The model under review builds one solid part; all positions refer to its coordinate system, in mm. Face numbers are marked on the shaded views. A direction names the side the tool comes from. Coordinates: 2 decimals unless noted, no trailing zeros. Loops run counter-clockwise (first coordinate to the right, second up) from the corner with the lowest first, then second, coordinate; pieces in that order, holes last. Notation, with made-up numbers: (80.25, 6) - (104.25, 6) arc R12 ccw to (104.25, 19) - close; hole circle Ø11 at (85, 54.25). An arc over 180 degrees is marked (long way). Use a Markdown table: item, result. Add a question column.
1) Add section D-D, the plane y = -65. Give the boundary of the cut face in (x, z).
2) The part is to be moulded in two halves that separate along Y. For the marked faces 1 and 2, say which applies: pulls with the +Y half, pulls with the -Y half, needs draft (parallel to the pull), parting line crosses it, or undercut.
3) To check wall thickness, follow L1, parallel to X at y = -77, z = -9.5; L2, parallel to Y at x = 200.5, z = -22; L3, parallel to Z at x = 25.5, y = -34.5. State the ranges of each line that lie inside material, in increasing order. Write a range as [from, to].
4) Clearance check with flat-ended pins moving along their axes: pin 1 (4 mm diameter, centred on x = 133.5, y = -2.5, fed in from -Z); pin 2 (3 mm diameter, centred on x = 21.5, y = -86.5, fed in from -Z); pin 3 (6 mm diameter, centred on x = 222.5, z = -70.5, fed in from +Y). State where each tip first meets the part, or that it passes through.
5) Add section C-C, the plane y = 85. Give the boundary of the cut face in (x, z).
6) Add section B-B, the plane x = 81. Give the boundary of the cut face in (y, z).
7) Add section A-A, the plane y = 0. Give the boundary of the cut face in (x, z).
8) For the marked faces 3 and 4, list the 3-axis set-ups (+Z, -Z, +X, -X, +Y, -Y) from which the entire face can be reached by the end or side of a thin tool; tool diameter is ignored.
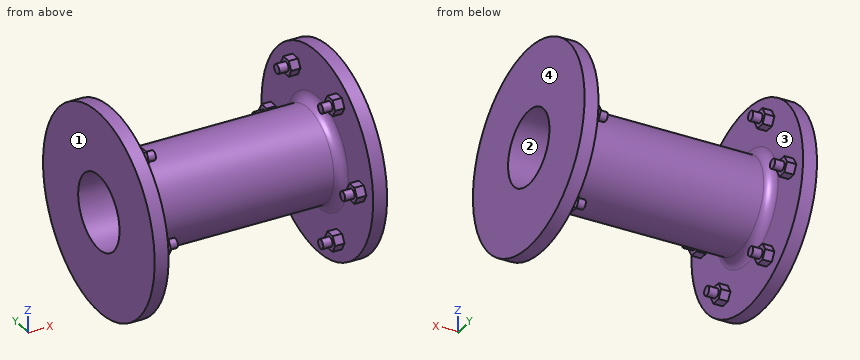
Autodesk Inventor part; units mm, degrees
ref_plane "YZ Plane" through (0, 0, 0) normal (1, 0, 0) x (0, 1, 0)
ref_plane "XZ Plane" through (0, 0, 0) normal (0, 1, 0) x (-1, 0, 0)
ref_plane "XY Plane" through (0, 0, 0) normal (0, 0, 1) x (1, 0, 0)
sketch "Skizze1" plane through (0, 0, 0) normal (1, 0, 0) x (0, 1, 0)
  circle A0 centre (0, 0) radius 40
  circle A1 centre (0, 0) radius 108
  dimension "d0" = 216
  dimension "d1" = 80
extrude "Extrusion1" add sketch "Skizze1" along normal blind 15
sketch "Skizze2" plane through (15, 0, 0) normal (1, 0, 0) x (0, 0, -1)
  circle A0 centre (0, 0) radius 40
  circle A1 centre (0, 0) radius 50
  dimension "d4" = 100
extrude "Extrusion2" add sketch "Skizze2" along normal blind 110
fillet "Rundung1" radius 10 1 edges at (15, 0, 50)
sketch "Skizze3" plane through (15, 0, 0) normal (1, 0, 0) x (0, 0, -1)
  circle A0 centre (0, -85) radius 10 construction
  line L0 (0, -95) -> (-8.7647, -89.8146)
  line L1 (-8.7647, -80.1854) -> (0, -75)
  line L2 (0, -75) -> (8.7647, -80.1854)
  line L3 (8.7647, -80.1854) -> (8.7647, -89.8146)
  line L4 (0, -95) -> (8.7647, -89.8146)
  line L5 (-8.7647, -80.1854) -> (-8.7647, -89.8146)
  point P0 (0, 0)
  dimension "d8" = 20
  dimension "d9" = 85
extrude "Extrusion3" add sketch "Skizze3" along normal blind 10
sketch "Skizze4" plane through (25, 0, 0) normal (1, 0, 0) x (0, 0, -1)
  circle A0 centre (0, -85) radius 5
  point P0 (0, 0)
  dimension "d12" = 10
extrude "Extrusion4" add sketch "Skizze4" along normal blind 10
pattern_circular "Runde Anordnung1" count 6 over 360 about axis through (-10, 0, 0) along (1, 0, 0) of "Extrusion3", "Extrusion4"
mirror "Spiegeln1" about plane through (125, 0, 0) normal (1, 0, 0) of "Extrusion3", "Extrusion4", "Runde Anordnung1", "Extrusion2", "Extrusion1", "Rundung1"
properties part number "DN80-025m"
From the geometry:
| question | item | result |
|---|---|---|
| 1 | outline | (0, -86.25) - (15, -86.25) - (15, 86.25) - (0, 86.25) - close; (235, -86.25) - (250, -86.25) - (250, 86.25) - (235, 86.25) - close |
| 2 | face 1 | needs draft |
| 2 | face 2 | undercut |
| 3 | L1 | x = [0, 15], [235, 250] |
| 3 | L2 | y = [-44.9, -33.41], [33.41, 44.9] |
| 3 | L3 | z = [-36.19, -20.24], [20.24, 36.19] |
| 4 | pin 1 | stops at z = -50 |
| 4 | pin 2 | stops at z = -8.76 |
| 4 | pin 3 | stops at y = 51.78 |
| 5 | outline | (0, -66.63) - (15, -66.63) - (15, -8.76) - (25, -8.76) - (25, -5) - (35, -5) - (35, 5) - (25, 5) - (25, 8.76) - (15, 8.76) - (15, 66.63) - (0, 66.63) - close; (215, -5) - (225, -5) - (225, -8.76) - (235, -8.76) - (235, -66.63) - (250, -66.63) - (250, 66.63) - (235, 66.63) - (235, 8.76) - (225, 8.76) - (225, 5) - (215, 5) - close |
| 6 | outline | circle Ø100 at (0, 0); hole circle Ø80 at (0, 0) |
| 7 | outline | (0, -108) - (15, -108) - (15, -60) arc R10 cw to (25, -50) - (225, -50) arc R10 cw to (235, -60) - (235, -108) - (250, -108) - (250, -40) - (0, -40) - close; (0, 40) - (250, 40) - (250, 108) - (235, 108) - (235, 60) arc R10 cw to (225, 50) - (25, 50) arc R10 cw to (15, 60) - (15, 108) - (0, 108) - close |
| 8 | face 3 | none |
| 8 | face 4 | +Z, -Z, +X, +Y, -Y |
